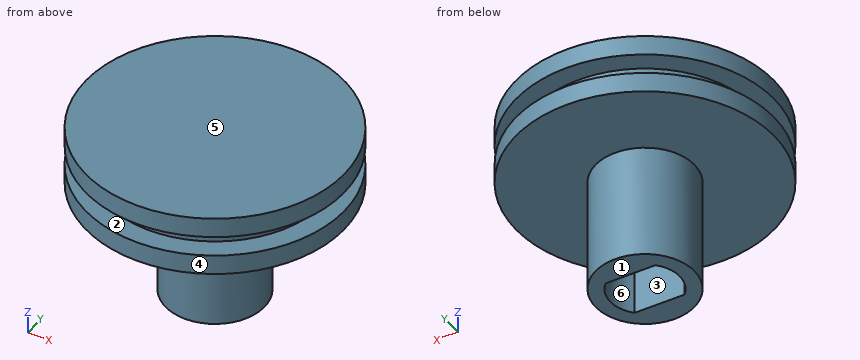
```python
from build123d import *

# Parameters (mm, degrees)
SKETCH1_R           = 3.725
BOSS_EXTRUDE1_DEPTH = 8.65
SKETCH2_R           = 9.725
BOSS_EXTRUDE2_DEPTH = 1.5
SKETCH3_R           = 8.225
BOSS_EXTRUDE3_DEPTH = 1.5
SKETCH5_R           = 9.725
BOSS_EXTRUDE5_DEPTH = 1.5


with BuildPart() as part:
    # Sketch1 → Boss-Extrude1 (new body)
    with BuildSketch(Plane.XY):
        with Locations(Location((0, 0, 0), (0, 0, 270))):
            Circle(SKETCH1_R)
        with BuildLine():
            Line((-1.886796226, -1.825), (1.886796226, -1.825))
            ThreePointArc((1.886796226, -1.825), (2.625, 0), (1.886796226, 1.825))
            Line((1.886796226, 1.825), (-1.886796226, 1.825))
            ThreePointArc((-1.886796226, 1.825), (-2.625, 0), (-1.886796226, -1.825))
        make_face(mode=Mode.SUBTRACT)
    extrude(amount=BOSS_EXTRUDE1_DEPTH)

    # Sketch2 → Boss-Extrude2 (add)
    with BuildSketch(Plane.XY.offset(8.65)):
        Circle(SKETCH2_R)
    extrude(amount=BOSS_EXTRUDE2_DEPTH)

    # Sketch3 → Boss-Extrude3 (add)
    with BuildSketch(Plane.XY.offset(10.15)):
        Circle(SKETCH3_R)
    extrude(amount=BOSS_EXTRUDE3_DEPTH)

    # Sketch5 → Boss-Extrude5 (add)
    with BuildSketch(Plane.XY.offset(11.65)):
        Circle(SKETCH5_R)
    extrude(amount=BOSS_EXTRUDE5_DEPTH)


solid = part.part
```
Can you work these out from the model? Positions are in its coordinate system, mm. Face numbers are marked on the shaded views. A direction names the side the tool comes from. Give positions to 0.01 mm unless a question says otherwise; leave off trailing zeros. Write each loop counter-clockwise with the first axis right and the second up, starting at its lowest first coordinate (ties: lowest second). Pieces come first, ordered by that corner, then holes. Notation, with made-up numbers: (79.5, -32) -> (91.5, -32) arc R35 ccw to (91.5, 5) -> close; hole circle Ø8 at (12.25, -31.5). An arc over 180 degrees is marked (long way). One line per item, written item: value.
Q1. Please list where these lines run through material, in increasing order: line 1 (Z direction, x = 6, y = -7.25); line 2 (Z direction, x = 2.5, y = 6.25); line 3 (X direction, y = -3.25, z = 6.5). Write a range as [from, to].
Results found:
line 1: z = [8.65, 10.15], [11.65, 13.15]
line 2: z = [8.65, 13.15]
line 3: x = [-1.82, 1.82]
Q2. Imagine slicing it at B-B on z = 1. Please give me the cut outline in (x, y) (3 decimals), and give its area (3 significant figures).
Results found:
outline: circle Ø7.45 at (0, 0); hole (-1.887, -1.825) -> (1.887, -1.825) arc R2.625 ccw to (1.887, 1.825) -> (-1.887, 1.825) arc R2.625 ccw to start
area: 26.1 mm^2
Q3. Which directions (+Z, -Z, +X, -X, +Y, -Y) give clear straight access to the entire face, cutting with the end or side of a thin tool? Please do the marked faces 1, 2 and 3.
Results found:
face 1: -Z, +X, -X, +Y, -Y
face 2: none
face 3: -Z
Q4. Imagine slicing it at C-C on y = 2.5. Please give me the cut outline in (x, z).
Results found:
outline: (-9.4, 8.65) -> (-2.76, 8.65) -> (-2.76, 0) -> (2.76, 0) -> (2.76, 8.65) -> (9.4, 8.65) -> (9.4, 10.15) -> (7.84, 10.15) -> (7.84, 11.65) -> (9.4, 11.65) -> (9.4, 13.15) -> (-9.4, 13.15) -> (-9.4, 11.65) -> (-7.84, 11.65) -> (-7.84, 10.15) -> (-9.4, 10.15) -> close
Q5. For P1, Ø3, axis at y = -5, z = 11.5, coming from the -X side; P2, Ø4, axis at x = 0, z = 4.5, coming from the -Y side (3 decimals); P3, Ø4, axis at x = 0, z = 3.5, coming from the +Y side (3 decimals); P4, Ø1, axis at y = 4.5, z = 8, coming from the +X side, each with a flat end and sliding along its axis, tell me the tip position at first contact or that it passes through.
Results found:
P1: stops at x = -9.07
P2: stops at y = -3.725
P3: stops at y = 3.725
P4: passes through
Q6. Imagine slicing it at D-D on z = 9. Please give me the cut outline in (x, y) (3 decimals).
Results found:
outline: circle Ø19.45 at (0, 0)
Q7. Imagine slicing it at A-A on x = 0. Please give me the cut outline in (y, z) (3 decimals).
Results found:
outline: (-9.725, 8.65) -> (-3.725, 8.65) -> (-3.725, 0) -> (-1.825, 0) -> (-1.825, 8.65) -> (1.825, 8.65) -> (1.825, 0) -> (3.725, 0) -> (3.725, 8.65) -> (9.725, 8.65) -> (9.725, 10.15) -> (8.225, 10.15) -> (8.225, 11.65) -> (9.725, 11.65) -> (9.725, 13.15) -> (-9.725, 13.15) -> (-9.725, 11.65) -> (-8.225, 11.65) -> (-8.225, 10.15) -> (-9.725, 10.15) -> close
Q8. We'd pull the mould along Y, two halves only. Please class the marked faces 4, 5 and 6: +Y half, -Y half, draft (parallel to the pull), parting line (faces both ways), or undercut.
Results found:
face 4: parting line
face 5: draft
face 6: undercut
